```python
from build123d import *

# Parameters (mm, degrees)
SKETCH1_W           = 59
SKETCH1_H           = 8
BOSS_EXTRUDE2_DEPTH = 75
FILLET1_R           = 37.5
SKETCH2_R           = 5
CUT_EXTRUDE1_DEPTH  = 10
SKETCH3_R           = 15
SKETCH3_R_2         = 5
BOSS_EXTRUDE3_DEPTH = 7.5
SKETCH4_R           = 10
SKETCH4_R_2         = 5
BOSS_EXTRUDE4_DEPTH = 7.5
SKETCH5_R           = 5
CUT_EXTRUDE2_DEPTH  = 10
SKETCH6_W           = 75
SKETCH6_H           = 35
BOSS_EXTRUDE5_DEPTH = 8
SKETCH7_W           = 59
SKETCH7_H           = 35
BOSS_EXTRUDE6_DEPTH = 8


with BuildPart() as part:
    # Sketch1 → Boss-Extrude2 (new body)
    with BuildSketch(Plane.XY):
        Polygon((8, -8), (8, -250), (0, -250), (0, 0), (75, 0), (75, -250), (67, -250), (67, -8), align=None)
        with Locations((37.5, -125)):
            Rectangle(SKETCH1_W, SKETCH1_H)
    extrude(amount=BOSS_EXTRUDE2_DEPTH)

    # Fillet1
    fillet1_edges = [part.edges().sort_by_distance(p)[0] for p in [
        (4, -250, 0),
        (71, -250, 0),
        (71, -250, 75),
        (4, -250, 75),
    ]]
    fillet(fillet1_edges, radius=FILLET1_R - 0.0001)  # a hair under: the kernel refuses the full size

    # Sketch2 → Cut-Extrude1 (cut)
    with BuildSketch(Plane(origin=(75, 0, 0), x_dir=(0, 0, -1), z_dir=(1, 0, 0))):
        with Locations(Location((-37.5, -212.5, 0), (0, 0, 90))):
            Circle(SKETCH2_R)
    extrude(amount=-CUT_EXTRUDE1_DEPTH, mode=Mode.SUBTRACT)

    # Sketch3 → Boss-Extrude3 (add)
    with BuildSketch(Plane.ZY.offset(-67)):
        with Locations(Location((37.5, -212.5, 0), (0, 0, 90))):
            Circle(SKETCH3_R)
        with Locations(Location((37.5, -212.5, 0), (0, 0, 90))):
            Circle(SKETCH3_R_2, mode=Mode.SUBTRACT)
    extrude(amount=BOSS_EXTRUDE3_DEPTH)

    # Sketch4 → Boss-Extrude4 (add)
    with BuildSketch(Plane.ZY.offset(-59.5)):
        with Locations(Location((37.5, -212.5, 0), (0, 0, 270))):
            Circle(SKETCH4_R)
        with Locations(Location((37.5, -212.5, 0), (0, 0, 90))):
            Circle(SKETCH4_R_2, mode=Mode.SUBTRACT)
    extrude(amount=BOSS_EXTRUDE4_DEPTH)

    # Sketch5 → Cut-Extrude2 (cut)
    with BuildSketch(Plane(origin=(0, 0, 0), x_dir=(1, 0, 0), z_dir=(0, 1, 0))):
        with Locations(Location((37.5, -37.5, 0), (0, 0, 180))):
            Circle(SKETCH5_R)
    extrude(amount=-CUT_EXTRUDE2_DEPTH, mode=Mode.SUBTRACT)

    # Sketch6 → Boss-Extrude5 (add)
    with BuildSketch(Plane(origin=(0, 0, 0), x_dir=(-1, 0, 0), z_dir=(0, 0, -1))):
        with Locations((-37.5, -83.5)):
            Rectangle(SKETCH6_W, SKETCH6_H)
        with Locations((-37.5, -166.5)):
            Rectangle(SKETCH6_W, SKETCH6_H)
    extrude(amount=-BOSS_EXTRUDE5_DEPTH)

    # Sketch7 → Boss-Extrude6 (add)
    with BuildSketch(Plane.XY.offset(75)):
        with Locations((37.5, -83.5)):
            Rectangle(SKETCH7_W, SKETCH7_H)
        with Locations((37.5, -166.5)):
            Rectangle(SKETCH7_W, SKETCH7_H)
    extrude(amount=-BOSS_EXTRUDE6_DEPTH)


solid = part.part
```
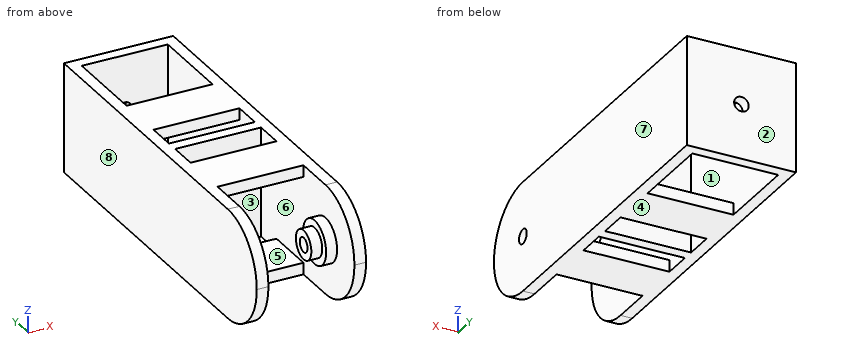
Input: part model. Units: mm. Frame: model coordinates. Face numbers are marked on the shaded views. A direction names the side the tool comes from. Coordinates: 2 decimals unless noted, no trailing zeros. Loops run counter-clockwise (first coordinate to the right, second up) from the corner with the lowest first, then second, coordinate; pieces in that order, holes last. Notation, with made-up numbers: M 12,-19.5 L 57,-19.5 A25 cw 57,19.5 Z; hole C -25,20 d8. An arc over 180 degrees is marked long. Use a Markdown table: item, result. Add a question column.
1) Line query: L1, parallel to Y at x = 26, z = 70; L2, parallel to Y at x = 63, z = 37; L3, parallel to X at y = -44, z = 6. Output: solid intervals per line, ascending. Write a range as from..to.
2) Section D-D, the plane z = 70. Return the cut outline in (x, y).
3) Section B-B, the plane y = -83. Return the cut outline in (x, z), plus the area to 3 significant figures.
4) Section A-A, the plane x = 18. Return the cut outline in (y, z), plus the area to 3 significant figures.
5) Section C-C, the plane x = 37.5. Return the cut outline in (y, z).
6) Pin query (flat end, axial travel): P1, Ø9, axis at x = 33, z = 5, coming from the -Y side; P2, Ø8, axis at x = 34, y = -106.5, coming from the -Z side. Return the tip coordinate at first contact, or that it passes through.
7) Set-up query: the marked faces 1, 2, 3, 4 and 5. Return all of +Z, -Z, +X, -X, +Y, -Y with unobstructed straight access to the full face (end or side cutting, diameter ignored); none if empty.
8) Draft query along X for the marked faces 6, 7 and 8. Return one class per face: +X half, -X half, draft (parallel to the pull), parting line (faces both ways), or undercut.
Answer below:
| question | item | result |
|---|---|---|
| 1 | L1 | -184..-149, -129..-121, -101..-66, -8..0 |
| 1 | L2 | -227.49..-217.47, -207.53..-197.51, -129..-121, -8..0 |
| 1 | L3 | 0..8, 67..75 |
| 2 | outline | M 0,-231.21 L 8,-231.21 L 8,-184 L 67,-184 L 67,-231.21 L 75,-231.21 L 75,0 L 0,0 Z; hole M 8,-149 L 67,-149 L 67,-129 L 8,-129 Z; hole M 8,-121 L 67,-121 L 67,-101 L 8,-101 Z; hole M 8,-66 L 67,-66 L 67,-8 L 8,-8 Z |
| 3 | outline | M 0,0 L 75,0 L 75,75 L 0,75 Z; hole M 8,8 L 67,8 L 67,67 L 8,67 Z |
| 3 | area | 2,140 mm2 |
| 4 | outline | M -184,0 L -149,0 L -149,8 L -184,8 Z; M -184,67 L -149,67 L -149,75 L -184,75 Z; M -129,0 L -121,0 L -121,75 L -129,75 Z; M -101,0 L -66,0 L -66,8 L -101,8 Z; M -101,67 L -66,67 L -66,75 L -101,75 Z; M -8,0 L 0,0 L 0,75 L -8,75 Z |
| 4 | area | 2,320 mm2 |
| 5 | outline | M -184,0 L -149,0 L -149,8 L -184,8 Z; M -184,67 L -149,67 L -149,75 L -184,75 Z; M -129,0 L -121,0 L -121,75 L -129,75 Z; M -101,0 L -66,0 L -66,8 L -101,8 Z; M -101,67 L -66,67 L -66,75 L -101,75 Z; M -8,0 L 0,0 L 0,32.5 L -8,32.5 Z; M -8,42.5 L 0,42.5 L 0,75 L -8,75 Z |
| 6 | P1 | y = -184 |
| 6 | P2 | through |
| 7 | face 1 | none |
| 7 | face 2 | +Z, -Z, +X, -X, +Y |
| 7 | face 3 | +Z, -Z |
| 7 | face 4 | -Z, +X, -X, +Y, -Y |
| 7 | face 5 | -Y |
| 8 | face 6 | undercut |
| 8 | face 7 | +X half |
| 8 | face 8 | -X half |
